The model under review builds one solid part; all positions refer to its coordinate system, in mm. Face numbers are marked on the shaded views. A direction names the side the tool comes from. Round coordinates to 2 decimals unless told otherwise and drop trailing zeros. Order: outer loops, then holes, each group sorted by start corner. A loop starts at its lowest first (then second) coordinate and runs counter-clockwise, first axis right, second up.
1) Consider section A-A (x = 43). Give the boundary of the cut face in (y, z).
2) Consider section B-B (x = 3.5). Give the boundary of the cut face in (y, z).
3) Mouldability with a two-part tool opening along Z and no side actions: class the marked faces 1, 2 and 3 as pulls with the +Z half, pulls with the -Z half, needs draft (parallel to the pull), parting line crosses it, or undercut.
4) Machinability: for the marked faces 4, 5, 6 and 7, which of the approach directions +Z, -Z, +X, -X, +Y, -Y give a long, thin tool a straight path to every point of the face, cutting with its end or side? Answer none if there is none.
5) Clearance check with flat-ended pins moving along their axes: P1, Ø4, axis at x = 40, z = 35.5, coming from the +Y side; P2, Ø7.5, axis at x = 26, y = 3, coming from the -Z side; P3, Ø6, axis at y = 77.5, z = -1.5, coming from the -X side. State where each tip first meets the part, or that it passes through.
6) Consider section C-C (z = 24). Give the boundary of the cut face in (x, y).
7) Consider section D-D (y = 70). Give the boundary of the cut face in (x, z), then the cut area to 3 significant figures.
8) To check wall thickness, follow L1, parallel to X at y = 36.5, z = 16; L2, parallel to Z at x = 40.5, y = 81; L3, parallel to Y at x = 43.5, z = 29. State the ranges of each line that lie inside material, in increasing order.
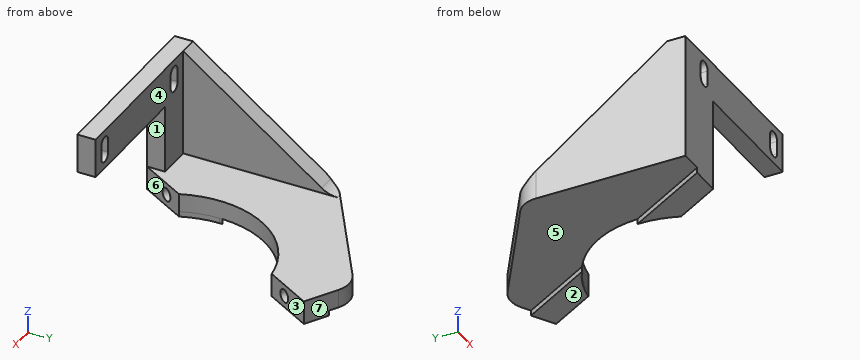
from build123d import *

# Parameters (mm, degrees)
BOSS_EXTRUDE1_DEPTH             = 7
BOSS_EXTRUDE3_DEPTH             = 2
TAP_DRILL_FOR_M6X1_0_TAP1_D     = 5
TAP_DRILL_FOR_M6X1_0_TAP1_DEPTH = 8
TAP_DRILL_FOR_M6X1_0_TAP1_TIP   = 1.502151548
BOSS_EXTRUDE4_DEPTH             = 7
BOSS_EXTRUDE5_DEPTH             = 7
SKETCH11_R                      = 2.5
CUT_EXTRUDE1_DEPTH              = 116.367305777
FILLET2_R                       = 10


with BuildPart() as part:
    # Sketch1 → Boss-Extrude1 (new body)
    with BuildSketch(Plane.XY):
        with BuildLine():
            Line((49.772581584, 68.888132052), (60, 86.602540378))
            Line((60, 86.602540378), (42.679491924, 96.602540378))
            Line((42.679491924, 96.602540378), (-10, 62.664913519))
            Line((-10, 62.664913519), (-10, 0))
            Line((-10, 0), (10, 0))
            Line((10, 0), (20.227418416, 17.714408326))
            ThreePointArc((20.227418416, 17.714408326), (22.524047358, 50.504264805), (49.772581584, 68.888132052))
        make_face()
    extrude(amount=-BOSS_EXTRUDE1_DEPTH)

    # Sketch5 → Boss-Extrude3 (add)
    with BuildSketch(Plane(origin=(0, 0, -7), x_dir=(-1, 0, 0), z_dir=(0, 0, -1))):
        with BuildLine():
            Line((-51.339745962, 91.602540378), (-60, 86.602540378))
            Line((-60, 86.602540378), (-49.772581584, 68.888132052))
            ThreePointArc((-49.772581584, 68.888132052), (-42.186769591, 66.997294279), (-35.157858732, 63.574689534))
            Line((-35.157858732, 63.574689534), (-51.339745962, 91.602540378))
        make_face()
        with BuildLine():
            ThreePointArc((-17.5, 31.754264805), (-18.188168957, 24.60310439), (-20.227418416, 17.714408326))
            Line((-20.227418416, 17.714408326), (-10, 0))
            Line((-10, 0), (1.547005384, 0))
            Line((1.547005384, 0), (-17.521633192, 33.027850844))
            ThreePointArc((-17.521633192, 33.027850844), (-17.505408688, 32.391149684), (-17.5, 31.754264805))
        make_face()
    extrude(amount=BOSS_EXTRUDE3_DEPTH)

    # Tap Drill for M6x1.0 Tap1
    with Locations(Plane(origin=(7.5, -4.330127019, 0), x_dir=(0, 0, -1), z_dir=(0.8660254037844368, -0.5000000000000031, 0))):
        with Locations((4.5, 92.5), (4.5, 17.5)):
            Hole(TAP_DRILL_FOR_M6X1_0_TAP1_D / 2, depth=TAP_DRILL_FOR_M6X1_0_TAP1_DEPTH)
            with Locations((0, 0, -(TAP_DRILL_FOR_M6X1_0_TAP1_DEPTH + TAP_DRILL_FOR_M6X1_0_TAP1_TIP / 2))):  # 118° drill point
                Cone(0, TAP_DRILL_FOR_M6X1_0_TAP1_D / 2, TAP_DRILL_FOR_M6X1_0_TAP1_TIP, mode=Mode.SUBTRACT)

    # Sketch9 → Boss-Extrude4 (add)
    with BuildSketch(Plane(origin=(0, 0, 0), x_dir=(1, 0, 0), z_dir=(0, 1, 0))):
        Polygon((-10, 0), (-10, -41), (60, -41), (60, -26), (10, -26), (10, 0), align=None)
    extrude(amount=BOSS_EXTRUDE4_DEPTH)

    # Sketch10 → Boss-Extrude5 (add)
    with BuildSketch(Plane.ZY.offset(10)):
        Polygon((0, 62.664913519), (41, 7), (0, 7), align=None)
    extrude(amount=-BOSS_EXTRUDE5_DEPTH)

    # Sketch11 → Cut-Extrude1 (cut, through all)
    with BuildSketch(Plane(origin=(0, 7, 0), x_dir=(1, 0, 0), z_dir=(0, 1, 0))):
        with Locations((3.5, -31)):
            Circle(SKETCH11_R)
        with BuildLine():
            ThreePointArc((3.5, -33.5), (5.267766953, -34.232233047), (6, -36))
            Line((6, -36), (6, -31))
            ThreePointArc((6, -31), (5.267766953, -32.767766953), (3.5, -33.5))
        make_face()
        with Locations((3.5, -36)):
            Circle(SKETCH11_R)
        with BuildLine():
            Line((1, -31), (1, -36))
            ThreePointArc((1, -36), (1.732233047, -34.232233047), (3.5, -33.5))
            ThreePointArc((3.5, -33.5), (1.732233047, -32.767766953), (1, -31))
        make_face()
        with Locations((53.5, -31)):
            Circle(SKETCH11_R)
        with Locations((53.5, -36)):
            Circle(SKETCH11_R)
        with BuildLine():
            Line((56, -36), (56, -31))
            ThreePointArc((56, -31), (55.267766953, -32.767766953), (53.5, -33.5))
            ThreePointArc((53.5, -33.5), (55.267766953, -34.232233047), (56, -36))
        make_face()
        with BuildLine():
            ThreePointArc((53.5, -33.5), (51.732233047, -32.767766953), (51, -31))
            Line((51, -31), (51, -36))
            ThreePointArc((51, -36), (51.732233047, -34.232233047), (53.5, -33.5))
        make_face()
    extrude(amount=-CUT_EXTRUDE1_DEPTH, mode=Mode.SUBTRACT)

    # Fillet2
    fillet2_edges = [part.edges().sort_by_distance(p)[0] for p in [
        (-6.5, 62.664913519, 0),
    ]]
    fillet(fillet2_edges, radius=FILLET2_R)
    fillet2_2_edges = [part.edges().sort_by_distance(p)[0] for p in [
        (-10, 62.664913519, -3.222472691),
        (42.679491924, 96.602540378, -3.5),
    ]]
    fillet(fillet2_2_edges, radius=FILLET2_R)


solid = part.part
Answer below:
1. outline: (0, 26) - (7, 26) - (7, 41) - (0, 41) - close; (67.28, -9) - (77.16, -9) - (77.16, -7) - (94.89, -7) - (94.89, 0) - (67.28, 0) - close
2. outline: (0, -9) - (8.74, -9) - (8.74, -7) - (71.36, -7) - (71.36, 0) - (7, 0) - (7, 28.5) - (0, 28.5) - close; (0, 38.5) - (7, 38.5) - (7, 41) - (0, 41) - close
3. face 1: undercut
3. face 2: pulls with the -Z half
3. face 3: needs draft
4. face 4: +Z, +X, +Y
4. face 5: -Z, -X, +Y
4. face 6: -Z, +X, -Y
4. face 7: +Z, -Z, +X, +Y
5. P1: stops at y = 7
5. P2: stops at z = 26
5. P3: stops at x = 8.37
6. outline: (-10, 0) - (10, 0) - (10, 7) - (-3, 7) - (-3, 30.08) - (-10, 30.08) - close
7. outline: (1.39, -7) - (38.87, -7) - (38.87, -9) - (50.41, -9) - (50.41, 0) - (1.39, 0) - close
7. area: 366 mm2
8. L1: x = -10 to -3
8. L2: z = -7 to 0
8. L3: y = 0 to 7
